Geometry check sheet. Reference: drawing and pictorial views, mm from the part's lowest x, y, z. A direction names the side the tool comes from. Coordinates: 2 decimals unless noted, no trailing zeros. Loops run counter-clockwise (first coordinate to the right, second up) from the corner with the lowest first, then second, coordinate; pieces in that order, holes last. Notation, with made-up numbers: (66.5, 17.5) - (72.5, 17.5) arc R19 ccw to (72.5, 52.5) - close; hole circle Ø3 at (16.5, 9). An arc over 180 degrees is marked (long way). Use a Markdown table: item, result. Add a question column.
1) Sectioned sample at C-C, the plane y = 20. Enter the section's corners in (x, z).
2) Thickness scan on line 1 (Y direction, x = 12, z = 0.9); line 2 (X direction, y = 10, z = 2.15); line 3 (X direction, y = 28, z = 3.5). Record the ranges inside material, lowest first.
3) Draft check along X on the marked faces 5 and 6. Enter one of: pulls with the +X half, pulls with the -X half, needs draft (parallel to the pull), parting line crosses it, or undercut.
4) Go/stop test with flat-tipped pins: P1, Ø1.6, axis at y = 36.5, z = 1, coming from the +X side; P2, Ø2, axis at x = 43.5, z = 3.5, coming from the -Y side; P3, Ø1.2, axis at x = 4, z = 1, coming from the +Y side. Record where each tip stops, or that it passes through.
5) Sectioned sample at A-A, the plane z = 2.9. Enter the section's corners in (x, y).
6) Sectioned sample at D-D, the plane x = 12. Enter the section's corners in (y, z).
7) Tool access check on the marked faces 1, 2, 3 and 4. Record the directions out of +Z, -Z, +X, -X, +Y, -Y that give a thin tool (end or side, any length) a straight path to the whole face; none if there is none.
8) Sectioned sample at B-B, the plane x = 27.5. Enter the section's corners in (y, z).
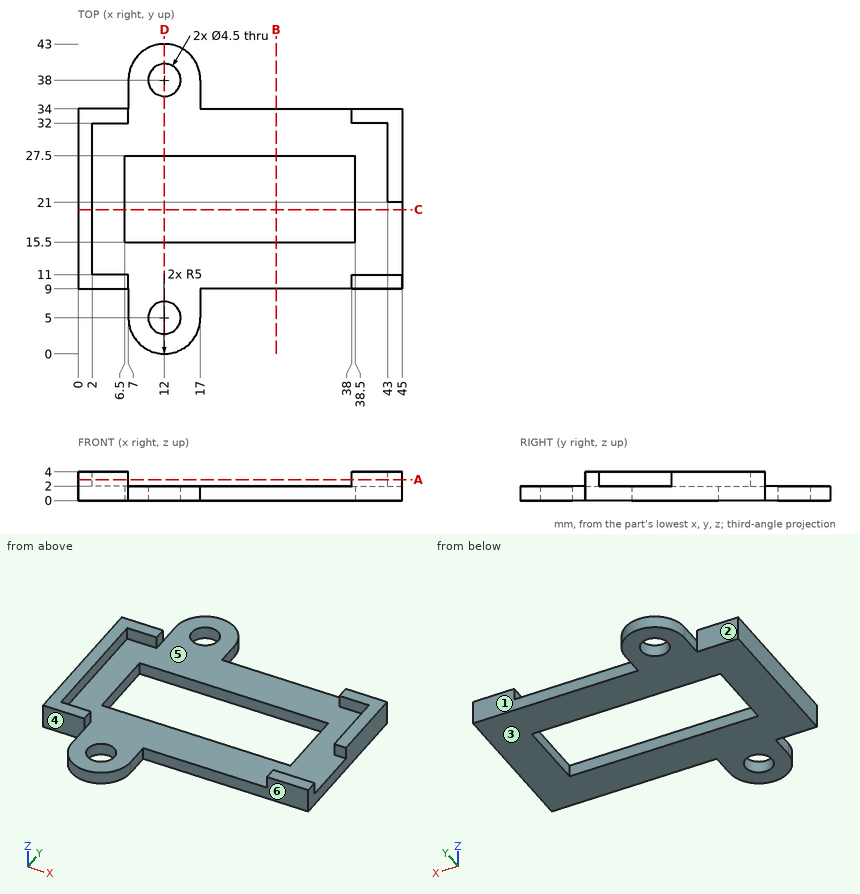
Solved:
| question | item | result |
|---|---|---|
| 1 | outline | (0, 0) - (6.5, 0) - (6.5, 2) - (2, 2) - (2, 4) - (0, 4) - close; (38.5, 0) - (45, 0) - (45, 2) - (38.5, 2) - close |
| 2 | line 1 | y = 0 to 2.75, 7.25 to 15.5, 27.5 to 35.75, 40.25 to 43 |
| 2 | line 2 | x = 0 to 7, 38 to 45 |
| 2 | line 3 | x = 0 to 2, 43 to 45 |
| 3 | face 5 | undercut |
| 3 | face 6 | needs draft |
| 4 | P1 | stops at x = 17 |
| 4 | P2 | stops at y = 9 |
| 4 | P3 | stops at y = 34 |
| 5 | outline | (0, 9) - (7, 9) - (7, 11) - (2, 11) - (2, 32) - (7, 32) - (7, 34) - (0, 34) - close; (38, 9) - (45, 9) - (45, 11) - (38, 11) - close; (38, 32) - (43, 32) - (43, 21) - (45, 21) - (45, 34) - (38, 34) - close |
| 6 | outline | (0, 0) - (2.75, 0) - (2.75, 2) - (0, 2) - close; (7.25, 0) - (15.5, 0) - (15.5, 2) - (7.25, 2) - close; (27.5, 0) - (35.75, 0) - (35.75, 2) - (27.5, 2) - close; (40.25, 0) - (43, 0) - (43, 2) - (40.25, 2) - close |
| 7 | face 1 | +Z, -Z, +X, +Y |
| 7 | face 2 | +Z, -Z, -X, +Y |
| 7 | face 3 | -Z, +X, -X, +Y, -Y |
| 7 | face 4 | +Z, -Z, -X, -Y |
| 8 | outline | (9, 0) - (15.5, 0) - (15.5, 2) - (9, 2) - close; (27.5, 0) - (34, 0) - (34, 2) - (27.5, 2) - close |
